Autodesk Inventor part; units mm, degrees
ref_plane "YZ Plane" through (0, 0, 0) normal (1, 0, 0) x (0, 1, 0)
ref_plane "XZ Plane" through (0, 0, 0) normal (0, 1, 0) x (-1, 0, 0)
ref_plane "XY Plane" through (0, 0, 0) normal (0, 0, 1) x (1, 0, 0)
sketch "Sketch1" plane through (0, 0, 0) normal (0, 0, 1) x (1, 0, 0)
  line L0 (0, 0) -> (140, 0) construction
  line L1 (140, 0) -> (140, 310) construction
  line L2 (140, 310) -> (0, 310) construction
  line L3 (0, 310) -> (0, 0) construction
  line L4 (15, 295) -> (125, 295) construction
  line L5 (125, 295) -> (125, 15) construction
  line L6 (125, 15) -> (15, 15) construction
  line L7 (15, 15) -> (15, 295) construction
  line L8 (15, 295) -> (125, 295) construction
  line L9 (70, 314.0975) -> (70, 322.6254) construction
  line L10 (15, 295) -> (15, 269.8596) construction
  line L11 (125, 295) -> (125, 292.6022) construction
  line L12 (0, 165.5) -> (-18, 165.5) construction
  line L13 (-18, 165.5) -> (-18, 185.5) construction
  line L14 (-18, 185.5) -> (0, 185.5) construction
  line L15 (0, 185.5) -> (0, 165.5) construction
  line L16 (-24.3067, 155) -> (-34.4998, 155) construction
  circle A0 centre (-9, 175.5) radius 3 construction
  line L17 (-18, 185.5) -> (0, 205.5) construction
  line L18 (0, 144.5) -> (-18, 144.5) construction
  line L19 (-18, 144.5) -> (-18, 124.5) construction
  circle A1 centre (-9, 134.5) radius 3 construction
  line L20 (-18, 124.5) -> (0, 104.5) construction
  line L21 (140, 165.5) -> (158, 165.5) construction
  line L22 (158, 165.5) -> (158, 185.5) construction
  circle A2 centre (149, 175.5) radius 3 construction
  line L23 (158, 185.5) -> (140, 205.5) construction
  line L24 (158, 144.5) -> (158, 124.5) construction
  line L25 (140, 144.5) -> (158, 144.5) construction
  circle A3 centre (149, 134.5) radius 3 construction
  line L26 (158, 124.5) -> (140, 104.5) construction
  line L27 (0, 300.2843) -> (9.7157, 310) construction
  line L28 (140, 300.2843) -> (130.2843, 310) construction
  line L29 (0, 9.7157) -> (9.7157, 0) construction
  line L30 (140, 9.7157) -> (130.2843, 0) construction
  line L31 (70, 295) -> (70, 310) construction
  line L32 (0, 155) -> (15, 155) construction
  line L33 (23.9173, 286.0827) -> (15, 295) construction
  line L34 (16.5096, 292.7523) -> (17.2477, 293.4904) construction
  line L35 (23.9173, 286.0827) -> (16.8787, 293.1213) construction
  line L36 (123.4904, 292.7523) -> (122.7523, 293.4904) construction
  line L37 (15, 17.2679) -> (15, 136.2679) construction
  arc A4 (14, 16.2679) -> (15, 17.2679) centre (14, 17.2679) ccw construction
  line L38 (14, 16.2679) -> (12, 16.2679) construction
  arc A5 (17, 17.2679) -> (18, 16.2679) centre (18, 17.2679) ccw construction
  spline S0 degree 3 poles (123.4904, 292.7523) (126.7806, 289.462) (122.6845, 284.0803) (122.5, 267.9145) knots 0 0 0 0 1 1 1 1 construction
  line L39 (15.2393, 288.9289) -> (15.2393, 218.384) construction
  line L40 (125, 148.5289) -> (125, 140.8711) construction
  line L41 (-110.1015, 148.4668) -> (-137.337, 121.2312) construction
  line L42 (-137.337, 121.2312) -> (-99.9418, 121.2312) construction
  line L43 (209.7417, 198.7679) -> (209.7417, 184.7679) construction
  line L44 (15, 148.5289) -> (15, 140.2675) construction
  line L45 (125, 148.5289) -> (125, 140.2675) construction
  spline S1 degree 4 poles (17.2477, 293.4904) (18.1955, 294.4381) (19.6714, 295.0826) (20.7017, 295) (21.8623, 295) knots 0 0 0 0 0 1 1 1 1 1 construction
  spline S2 degree 3 poles (122.7523, 293.4904) (121.4886, 294.7541) (119.4432, 295.1927) (118.1377, 295) knots 0 0 0 0 1 1 1 1 construction
  line L46 (118.1377, 295) -> (21.8623, 295) construction
  line L47 (16.8787, 293.1213) -> (23.2316, 286.7684) construction
  arc A6 (19, 310) -> (0, 291) centre (19, 291) ccw construction
  arc A7 (19, 295) -> (15, 291) centre (19, 291) ccw construction
  line L48 (19, 291) -> (10, 291) construction
  line L49 (19, 291) -> (19, 300) construction
  line L50 (16.1716, 293.8284) -> (5.565, 304.435) construction
  circle A8 centre (10.8683, 299.1317) radius 2 construction
  line L51 (9.8231, 300.915) -> (9.085, 300.1769) construction
  line L52 (11.9134, 297.3485) -> (12.6515, 298.0866) construction
  circle A9 centre (70, 302.5) radius 2 construction
  circle A10 centre (7.5, 155) radius 2 construction
  circle A11 centre (7.5, 227.0659) radius 2 construction
  line L53 (7.5, 155) -> (7.5, 227.0659) construction
  line L54 (7.5, 227.0659) -> (7.5, 299.1317) construction
  arc A12 (140, 291) -> (121, 310) centre (121, 291) ccw construction
  arc A13 (125, 291) -> (121, 295) centre (121, 291) ccw construction
  circle A14 centre (129.1317, 299.1317) radius 2 construction
  circle A15 centre (132.5, 155) radius 2 construction
  circle A16 centre (132.5, 227.0659) radius 2 construction
  circle A17 centre (10.8683, 10.8683) radius 2 construction
  circle A18 centre (70, 7.5) radius 2 construction
  circle A19 centre (7.5, 82.9341) radius 2 construction
  circle A20 centre (132.5, 82.9341) radius 2 construction
  circle A21 centre (129.1317, 10.8683) radius 2 construction
  arc A22 (0, 19) -> (19, 0) centre (19, 19) ccw construction
  arc A23 (15, 19) -> (19, 15) centre (19, 19) ccw construction
  arc A24 (121, 0) -> (140, 19) centre (121, 19) ccw construction
  arc A25 (121, 15) -> (125, 19) centre (121, 19) ccw construction
  circle A26 centre (10.8683, 299.1317) radius 7.5 construction
  line L55 (4.4716, 303.3416) -> (6.8718, 305.7419) construction
  line L56 (15, 140.2675) -> (15, 136.2679) construction
  line L57 (125, 138.6822) -> (125, 140.2675) construction
  line L58 (15, 138.6822) -> (15, 140.2675) construction
  line L59 (19, 15) -> (121, 15) construction
  line L60 (121, 0) -> (19, 0) construction
  line L61 (15, 291) -> (15, 19) construction
  line L62 (0, 19) -> (0, 291) construction
  line L63 (125, 291) -> (125, 19) construction
  line L64 (140, 19) -> (140, 291) construction
  line L65 (19, 295) -> (121, 295) construction
  line L66 (121, 310) -> (19, 310) construction
  arc A27 (132.5, 291) -> (121, 302.5) centre (121, 291) ccw construction
  arc A28 (139.5, 291) -> (121, 309.5) centre (121, 291) ccw
  arc A29 (125.5, 291) -> (121, 295.5) centre (121, 291) ccw
  arc A30 (125.5, 291) -> (139.5, 291) centre (132.5, 291) ccw construction
  arc A31 (121, 309.5) -> (121, 295.5) centre (121, 302.5) ccw construction
  arc A32 (19, 309.5) -> (0.5, 291) centre (19, 291) ccw
  arc A33 (19, 295.5) -> (14.5, 291) centre (19, 291) ccw
  arc A34 (121, 0.5) -> (139.5, 19) centre (121, 19) ccw
  arc A35 (121, 14.5) -> (125.5, 19) centre (121, 19) ccw
  arc A36 (14.5, 19) -> (19, 14.5) centre (19, 19) ccw
  arc A37 (0.5, 19) -> (19, 0.5) centre (19, 19) ccw
  line L67 (139.5, 19) -> (139.5, 291)
  line L68 (125.5, 291) -> (125.5, 19)
  line L69 (121, 14.5) -> (19, 14.5)
  line L70 (19, 0.5) -> (121, 0.5)
  line L71 (14.5, 19) -> (14.5, 291)
  line L72 (0.5, 291) -> (0.5, 19)
  line L73 (121, 295.5) -> (19, 295.5)
  line L74 (19, 309.5) -> (121, 309.5)
  point P0 (70, 318.3615)
  point P1 (-29.4032, 155)
  point P2 (-18, 175.5)
  point P3 (-9, 185.5)
  point P4 (124.7607, 288.9289)
  point P5 (209.7417, 191.7679)
  point P6 (19.6961, 294.835)
  point P7 (120.3039, 294.835)
  point P8 (9.4541, 300.5459)
  point P9 (12.2825, 297.7175)
  dimension "d163" = 4
  dimension "d0" = 140
  dimension "d1" = 310
  dimension "d2" = 15
  dimension "d85" = 18
  dimension "d86" = 20
  dimension "d87" = 10.5
  dimension "d88" = 6
  dimension "d89" = 20
  dimension "d114" = 135
  dimension "d126" = 1
  dimension "d128" = 2
  dimension "d152" = 45
  dimension "d158" = 45
  dimension "d161" = 4
  dimension "d164" = 5.5
  dimension "d168" = 15
  dimension "d169" = 1
  dimension "d170" = 1
  dimension "d171" = 1
  dimension "expansion" = 0.5
  dimension "d201" = 0.5
extrude "Extrusion7" add sketch "Sketch1" along normal blind 0.5
hole "Hole1" at (129.1317, 299.1317, 0) at (70, 302.5, 0) at (10.8683, 299.1317, 0) at (7.5, 227.0659, 0) at (132.5, 227.0659, 0) at (132.5, 155, 0) at (7.5, 155, 0) at (132.5, 82.9341, 0) at (129.1317, 10.8683, 0) at (70, 7.5, 0) at (10.8683, 10.8683, 0) at (7.5, 82.9341, 0) direction (0, 0, 1) diameter 4.1 end through all
properties part number "GB-gasket"
The model under review builds one solid part; all positions refer to its coordinate system, in mm. Round coordinates to 2 decimals unless told otherwise and drop trailing zeros. Write each loop counter-clockwise with the first axis right and the second up, starting at its lowest first coordinate (ties: lowest second). Pieces come first, ordered by that corner, then holes. Notation, with made-up numbers: (68.25, 0) - (103.25, 0) arc R16 cw to (103.25, 30) - close; hole circle Ø7 at (-20.75, 35.5). An arc over 180 degrees is marked (long way). One line per item, written item: value. Start each with the question number.
1. Consider section A-A on y = 198.5. Write out the cut boundary in (x, z).
2. To check wall thickness, follow L1, parallel to Y at x = 70, z = 0.25; L2, parallel to Y at x = 45.5, z = 0.4; L3, parallel to X at y = 192, z = 0.1. State the ranges of each line that lie inside material, in increasing order. Write a range as from..to.
3. Clearance check with flat-ended pins moving along their axes: P1, Ø3.5, axis at x = 7.5, y = 155, coming from the +Z side; P2, Ø6.5, axis at x = 10.87, y = 10.87, coming from the -Z side. State where each tip first meets the part, or that it passes through.
4. Consider section B-B on x = 80. Write out the cut boundary in (y, z).
5. Consider section C-C on z = 0.35. State how many separate pieces and enclosed holes the cut face has, and give its area (3 significant figures).
Checks:
1. outline: (0.5, 0) - (14.5, 0) - (14.5, 0.5) - (0.5, 0.5) - close; (125.5, 0) - (139.5, 0) - (139.5, 0.5) - (125.5, 0.5) - close
2. L1: y = 0.5..5.45, 9.55..14.5, 295.5..300.45, 304.55..309.5
2. L2: y = 0.5..14.5, 295.5..309.5
2. L3: x = 0.5..14.5, 125.5..139.5
3. P1: passes through
3. P2: stops at z = 0
4. outline: (0.5, 0) - (14.5, 0) - (14.5, 0.5) - (0.5, 0.5) - close; (295.5, 0) - (309.5, 0) - (309.5, 0.5) - (295.5, 0.5) - close
5. separate pieces: 1
5. enclosed holes: 13
5. area: 11,300 mm^2
